The model under review builds one solid part; all positions refer to its coordinate system, in mm. A direction names the side the tool comes from. Coordinates: 2 decimals unless noted, no trailing zeros. Loops run counter-clockwise (first coordinate to the right, second up) from the corner with the lowest first, then second, coordinate; pieces in that order, holes last. Notation, with made-up numbers: M -16.75,13.5 L 1.25,13.5 A14 ccw 1.25,33.5 Z; hole C 28,47 d7. An arc over 180 degrees is marked long. Use CSV: the item, a comma, the result in double quotes. Start each with the question number.
1. Draft analysis for pull direction X (two halves, no side actions). For faces 4 (the flat face through (450, 197, -83)), 5 (the flat face through (197, 203, 0)), 6 (the flat face through (308, 204, -310)), state which applies: +X half, -X half, draft (parallel to the pull), parting line (faces both ways), or undercut.
2. Tool access review of faces 1 (the flat face through (197, -50, -83)), 2 (the flat face through (375, 203, -10)), 3 (the flat face through (300, 199, -167)): name each direction out of +Z, -Z, +X, -X, +Y, -Y from which nothing blocks a thin tool from reaching the whole face with its end or side.
3. Add section A-A, the plane z = -181. Write out the cut boundary in (x, y), then the cut area to 3 significant figures.
4. For L1, parallel to Z at x = 224.5, y = 334; L2, parallel to Z at x = 104.5, y = 363.5; L3, parallel to Y at x = 191.5, z = -236.5, list the stretches that pass through material, from the lowest coordinate up.
5. Add section B-B, the plane x = 43. Write out the cut boundary in (y, z).
6. Add section C-C, the plane y = 211.5. Write out the cut boundary in (x, z), then the cut area to 3 significant figures.
from build123d import *

# Parameters (mm, degrees)
BOX007_W     = 300
BOX007_H     = 300
BOX007_DEPTH = 10
BOX006_W     = 200
BOX006_H     = 200
BOX006_DEPTH = 300
BOX005_W     = 400
BOX005_H     = 400
BOX005_DEPTH = 300
BOX009_W     = 400
BOX009_H     = 400
BOX009_DEPTH = 410
BOX008_W     = 500
BOX008_H     = 500
BOX008_DEPTH = 460
BOX002_W     = 400
BOX002_H     = 400
BOX002_DEPTH = 100


with BuildPart() as cube006:
    # Box007 → Box007 (new body)
    with BuildSketch(Plane(origin=(50, 50, -20), x_dir=(1, 0, 0), z_dir=(0, 0, 1))):
        with Locations((150, 150)):
            Rectangle(BOX007_W, BOX007_H)
    extrude(amount=BOX007_DEPTH)


with BuildPart() as cube005:
    # Box006 → Box006 (new body)
    with BuildSketch(Plane(origin=(100, 100, -310), x_dir=(1, 0, 0), z_dir=(0, 0, 1))):
        with Locations((100, 100)):
            Rectangle(BOX006_W, BOX006_H)
    extrude(amount=BOX006_DEPTH)


with BuildPart() as cut003:
    # Box005 → Box005 (new body)
    with BuildSketch(Plane.XY.offset(-310)):
        with Locations((200, 200)):
            Rectangle(BOX005_W, BOX005_H)
    extrude(amount=BOX005_DEPTH)

    # Cut002: cut Cube005
    add(cube005.part, mode=Mode.SUBTRACT)

    # Cut003: cut Cube006
    add(cube006.part, mode=Mode.SUBTRACT)


with BuildPart() as cube008:
    # Box009 → Box009 (new body)
    with BuildSketch(Plane.XY.offset(-310)):
        with Locations((200, 200)):
            Rectangle(BOX009_W, BOX009_H)
    extrude(amount=BOX009_DEPTH)


with BuildPart() as cut004:
    # Box008 → Box008 (new body)
    with BuildSketch(Plane(origin=(-50, -50, -310), x_dir=(1, 0, 0), z_dir=(0, 0, 1))):
        with Locations((250, 250)):
            Rectangle(BOX008_W, BOX008_H)
    extrude(amount=BOX008_DEPTH)

    # Cut004: cut Cube008
    add(cube008.part, mode=Mode.SUBTRACT)


with BuildPart() as obj1:
    # Box002 → Box002 (new body)
    with BuildSketch(Plane.XY):
        with Locations((200, 200)):
            Rectangle(BOX002_W, BOX002_H)
    extrude(amount=BOX002_DEPTH)

    # Fusion001: union Cut003, Cut004
    add(cut003.part)
    add(cut004.part)


solid = obj1.part
Computed:
1,face 4,"+X half"
1,face 5,"undercut"
1,face 6,"draft"
2,face 1,"+Z, -Z, +X, -X, -Y"
2,face 2,"none"
2,face 3,"-Z"
3,outline,"M -50,-50 L 450,-50 L 450,450 L -50,450 Z; hole M 100,100 L 300,100 L 300,300 L 100,300 Z"
3,area,"210,000 mm^2"
4,L1,"z = -310 to -20, 0 to 150"
4,L2,"z = -310 to -10, 0 to 150"
4,L3,"y = -50 to 100, 300 to 450"
5,outline,"M -50,-310 L 450,-310 L 450,150 L -50,150 Z; hole M 0,-10 L 400,-10 L 400,0 L 0,0 Z"
6,outline,"M -50,-310 L 100,-310 L 100,-20 L 50,-20 L 50,-10 L 0,-10 L 0,0 L 400,0 L 400,-10 L 350,-10 L 350,-20 L 300,-20 L 300,-310 L 450,-310 L 450,150 L -50,150 Z"
6,area,"165,000 mm^2"
